Model file for the job. Use its own axes, mm. Face numbers are marked on the shaded views. A direction names the side the tool comes from. Give positions to 0.01 mm unless a question says otherwise; leave off trailing zeros. Write each loop counter-clockwise with the first axis right and the second up, starting at its lowest first coordinate (ties: lowest second). Pieces come first, ordered by that corner, then holes.
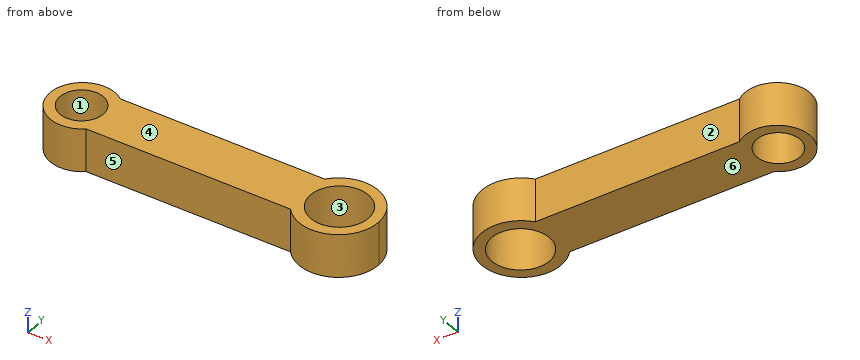
```python
from build123d import *

# Parameters (mm, degrees)
BOSS_EXTRUDE2_DEPTH      = 6
CUT_EXTRUDE1_OUTLINE_R   = 4
CUT_EXTRUDE1_OUTLINE_R_2 = 3
CUT_EXTRUDE1_DEPTH       = 6


# Read off the part's stored shape, not the designer's step: Cut-Extrude1
with BuildPart() as part:
    # Sketch1 → Boss-Extrude2 (new body)
    with BuildSketch(Plane.XY):
        with BuildLine():
            Line((-15.512, -3.5), (-15.512, 3.5))
            Line((-15.512, 3.5), (-14.027572875, 3.5))
            ThreePointArc((-14.027572875, 3.5), (-21.356, 0), (-14.027572875, -3.5))
            Line((-14.027572875, -3.5), (-15.512, -3.5))
        make_face()
        with BuildLine():
            Line((-14.027572875, 3.5), (-15.512, 3.5))
            Line((-15.512, 3.5), (-15.512, -3.5))
            Line((-15.512, -3.5), (-14.027572875, -3.5))
            ThreePointArc((-14.027572875, -3.5), (-12.795339828, -1.939339828), (-12.356, 0))
            ThreePointArc((-12.356, 0), (-12.795339828, 1.939339828), (-14.027572875, 3.5))
        make_face()
        with BuildLine():
            Line((13.901359313, 3.5), (-14.027572875, 3.5))
            ThreePointArc((-14.027572875, 3.5), (-12.795339828, 1.939339828), (-12.356, 0))
            ThreePointArc((-12.356, 0), (-12.795339828, -1.939339828), (-14.027572875, -3.5))
            Line((-14.027572875, -3.5), (13.901359313, -3.5))
            ThreePointArc((13.901359313, -3.5), (12.644, 0), (13.901359313, 3.5))
        make_face()
        with BuildLine():
            ThreePointArc((23.644, 0), (20.003499425, 5.176124215), (13.901359313, 3.5))
            Line((13.901359313, 3.5), (15.512, 3.5))
            Line((15.512, 3.5), (15.512, -3.5))
            Line((15.512, -3.5), (13.901359313, -3.5))
            ThreePointArc((13.901359313, -3.5), (20.003499425, -5.176124215), (23.644, 0))
        make_face()
        with BuildLine():
            Line((15.512, 3.5), (13.901359313, 3.5))
            ThreePointArc((13.901359313, 3.5), (12.644, 0), (13.901359313, -3.5))
            Line((13.901359313, -3.5), (15.512, -3.5))
            Line((15.512, -3.5), (15.512, 3.5))
        make_face()
    extrude(amount=BOSS_EXTRUDE2_DEPTH)

    # Cut-Extrude1 outline → Cut-Extrude1 (cut)
    with BuildSketch(Plane.XY):
        with Locations((18.253573905, 0)):
            Circle(CUT_EXTRUDE1_OUTLINE_R)
        with Locations((-16.991061145, 0)):
            Circle(CUT_EXTRUDE1_OUTLINE_R_2)
    extrude(amount=CUT_EXTRUDE1_DEPTH, mode=Mode.SUBTRACT)


solid = part.part
```
1. Probe probe 1 along X at (y, z) = (-2.5, 1.3); probe 2 along X at (y, z) = (2, 5.2) (3 decimals); probe 3 along Y at (x, z) = (11, 5.6). List the from-to ranges inside material, lowest first.
Calculated:
probe 1: x = -20.6 to -18.65, -15.33 to 15.13, 21.38 to 23.04
probe 2: x = -20.887 to -19.227, -14.755 to 14.789, 21.718 to 23.267
probe 3: y = -3.5 to 3.5
2. Slice it at A-A, the plane z = 5.2. Write the cut outline in (x, y).
Calculated:
outline: (-14.03, -3.5) - (13.9, -3.5) arc R5.5 ccw (long way) to (13.9, 3.5) - (-14.03, 3.5) arc R4.5 ccw (long way) to start; hole circle Ø6 at (-16.99, 0); hole circle Ø8 at (18.25, 0)
3. Which spindle directions (+Z, -Z, +X, -X, +Y, -Y) get a long thin tool onto all of the face, cutting with end or side? Do the marked faces 5 and 6. Say none if no direction does.
Calculated:
face 5: +Z, -Z, -Y
face 6: -Z, +X, -X, +Y, -Y
4. Slice it at D-D, the plane x = 13.5. Write the cut outline in (y, z).
Calculated:
outline: (-3.5, 0) - (3.5, 0) - (3.5, 6) - (-3.5, 6) - close
5. Pull direction Y, two halves, no side cores. Call the marked faces 1, 2, 3 and 4: +Y half, -Y half, draft (parallel to the pull), parting line (faces both ways), or undercut.
Calculated:
face 1: undercut
face 2: +Y half
face 3: undercut
face 4: draft
6. Slice it at B-B, the plane y = 2. Write the cut outline in (x, z) (3 decimals).
Calculated:
outline: (-20.887, 0) - (-19.227, 0) - (-19.227, 6) - (-20.887, 6) - close; (-14.755, 0) - (14.789, 0) - (14.789, 6) - (-14.755, 6) - close; (21.718, 0) - (23.267, 0) - (23.267, 6) - (21.718, 6) - close
7. Slice it at C-C, the plane x = -15. Write the cut outline in (y, z), and give its area (3 significant figures).
Calculated:
outline: (-4.1, 0) - (-2.24, 0) - (-2.24, 6) - (-4.1, 6) - close; (2.24, 0) - (4.1, 0) - (4.1, 6) - (2.24, 6) - close
area: 22.3 mm2
8. Pin check, flat tips, straight feed: P1, Ø1.5, axis at y = -1.5, z = 5, coming from the -X side; P2, Ø2, axis at x = -1.5, z = 1.5, coming from the -Y side; P3, Ø3, axis at y = 2.5, z = 3, coming from the -X side. Stop position of each tip, or through.
Calculated:
P1: stops at x = -21.29
P2: stops at y = -3.5
P3: stops at x = -21.24
